from build123d import *

# Parameters (mm, degrees)
SKETCH_1_W        = 55.5
SKETCH_1_H        = 35.5
EXTRUDE_764_DEPTH = 33
SKETCH_2_W        = 9
SKETCH_2_H        = 15
SKETCH_3_W        = 5.1
SKETCH_3_H        = 15
SKETCH_4_W        = 12
SKETCH_4_H        = 12
EXTRUDE_919_DEPTH = 31.6


with BuildPart() as part:
    # Sketch 1 → Extrude 764 (new, symmetric)
    with BuildSketch(Plane(origin=(0, 0, 0), x_dir=(0, 0, -1), z_dir=(1, 0, 0))):
        with Locations((9.65, 0)):
            Rectangle(SKETCH_1_W, SKETCH_1_H)
    extrude(amount=EXTRUDE_764_DEPTH, both=True)

    # Sketch 2 → Revolve 816 (revolve)
    with BuildSketch(Plane.XY, mode=Mode.PRIVATE) as revolve_816_sk:
        with Locations((37.5, 7.5)):
            Rectangle(SKETCH_2_W, SKETCH_2_H)
    revolve(revolve_816_sk.sketch.rotate(Axis((0, 0, 0), (1, 0, 0)), 90), axis=Axis((0, 0, 0), (1, 0, 0)))

    # Sketch 3 → Revolve 870 (revolve)
    with BuildSketch(Plane.XY, mode=Mode.PRIVATE) as revolve_870_sk:
        with Locations((-35.55, 7.5)):
            Rectangle(SKETCH_3_W, SKETCH_3_H)
    revolve(revolve_870_sk.sketch.rotate(Axis((0, 0, 0), (1, 0, 0)), 90), axis=Axis((0, 0, 0), (1, 0, 0)))

    # Sketch 4 → Extrude 919 (add, symmetric)
    with BuildSketch(Plane.XY):
        with Locations((18, 0)):
            Rectangle(SKETCH_4_W, SKETCH_4_H)
    extrude(amount=EXTRUDE_919_DEPTH, both=True)


solid = part.part
Could you check a few things on this model? Use its own coordinates, in mm. A direction names the side the tool comes from. Round coordinates to 2 decimals unless told otherwise and drop trailing zeros. Write each loop counter-clockwise with the first axis right and the second up, starting at its lowest first coordinate (ties: lowest second). Pieces come first, ordered by that corner, then holes. Notation, with made-up numbers: (-26.75, 75) - (1.25, 75) arc R11 cw to (1.25, 90) - close; hole circle Ø3 at (3.25, 77). An arc over 180 degrees is marked (long way). Put each result on its own line as item: value. Start each with the question number.
(1) I want a section at D-D, the plane z = 9. Please give me the cut outline in (x, y), plus the area to 3 significant figures.
(2) I want a section at B-B, the plane z = 0. Please give me the cut outline in (x, y).
(3) I want a section at C-C, the plane x = 22.5. Please give me the cut outline in (y, z).
(4) For faces 1 (the flat face through (24, 0, 25)), 2 (the flat face through (18, 6, 25)), 3 (the cylindrical face through (-35.51, -12.65, 8.06)), 4 (the flat face through (12, 0, 25)), 5 (the flat face through (18, -6, 25)), which set-ups out of +Z, -Z, +X, -X, +Y, -Y let a thin tool reach every point of the face, with its end or its side?
(5) I need wall thicknesses on probe 1 along X at (y, z) = (13.5, 8.5); probe 2 along Z at (x, y) = (-20.5, 8.5); probe 3 along X at (y, z) = (5.5, 28). Which ranges of each line are inside material? Lowest first, please.
(6) I want a section at A-A, the plane y = 0. Please give me the cut outline in (x, z).
(7) Will these pins go through, and if not, where does the flat tip stop? pin 1 (13 mm diameter, centred on x = 16, z = 25.5, fed in from +Y); pin 2 (13 mm diameter, centred on y = 1.5, z = 27.5, fed in from +X); pin 3 (13 mm diameter, centred on y = 1.5, z = 24.5, fed in from -X).
Here are the results:
1. outline: (-38.1, -12) - (-33, -12) - (-33, -17.75) - (33, -17.75) - (33, -12) - (42, -12) - (42, 12) - (33, 12) - (33, 17.75) - (-33, 17.75) - (-33, 12) - (-38.1, 12) - close
1. area: 2,680 mm^2
2. outline: (-38.1, -15) - (-33, -15) - (-33, -17.75) - (33, -17.75) - (33, -15) - (42, -15) - (42, 15) - (33, 15) - (33, 17.75) - (-33, 17.75) - (-33, 15) - (-38.1, 15) - close
3. outline: (-17.75, -37.4) - (17.75, -37.4) - (17.75, 18.1) - (6, 18.1) - (6, 31.6) - (-6, 31.6) - (-6, 18.1) - (-17.75, 18.1) - close
4. face 1: +Z, +X, +Y, -Y
4. face 2: +Z, +X, -X, +Y
4. face 3: -X
4. face 4: +Z, -X, +Y, -Y
4. face 5: +Z, +X, -X, -Y
5. probe 1: x = -33 to 33
5. probe 2: z = -37.4 to 18.1
5. probe 3: x = 12 to 24
6. outline: (-38.1, -15) - (-33, -15) - (-33, -37.4) - (33, -37.4) - (33, -15) - (42, -15) - (42, 15) - (33, 15) - (33, 18.1) - (24, 18.1) - (24, 31.6) - (12, 31.6) - (12, 18.1) - (-33, 18.1) - (-33, 15) - (-38.1, 15) - close
7. pin 1: stops at y = 6
7. pin 2: stops at x = 24
7. pin 3: stops at x = -33
